Job drawing, mm, ordinate dimensions from the low corner. One solid piece. A direction names the side the tool comes from. Round coordinates to 2 decimals unless told otherwise and drop trailing zeros. Write each loop counter-clockwise with the first axis right and the second up, starting at its lowest first coordinate (ties: lowest second). Pieces come first, ordered by that corner, then holes.
1) Pull direction Y, two halves, no side cores. Call the marked faces 1, 2 and 3: +Y half, -Y half, draft (parallel to the pull), parting line (faces both ways), or undercut.
2) Saw through at B-B (y = 15.5). Write the cut outline in (x, z) (1 decimal).
3) Flat gauge pins, fed straight in: pin 1 (1 mm diameter, centred on y = 21, z = 1, fed in from +X); pin 2 (3.5 mm diameter, centred on y = 12.5, z = 1.5, fed in from -X); pin 3 (1 mm diameter, centred on y = 14, z = 6.5, fed in from +X) (1 decimal). Where does each tip first touch, or does it go through?
4) Wall check: probe 1 along Z at (x, y) = (6, 22.5); probe 2 along X at (y, z) = (27.5, 2.25); probe 3 along Z at (x, y) = (2, 30) (1 decimal). Give the ranges that are in metal, low to high.
5) Saw through at A-A (z = 6). State how many separate pieces and enclosed holes the cut face has, plus the area to 3 significant figures.
6) Which spindle directions (+Z, -Z, +X, -X, +Y, -Y) get a long thin tool onto all of the face, cutting with end or side? Do the marked faces 4, 5, 6 and 7. Say none if no direction does.
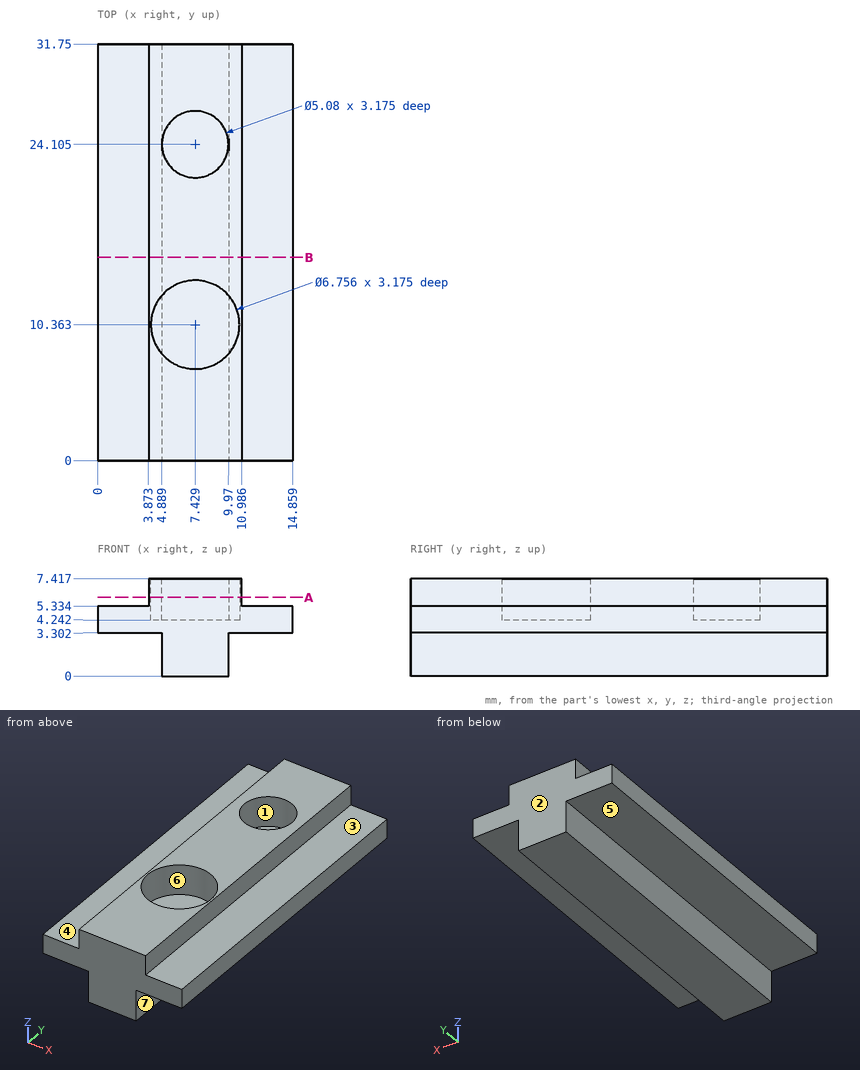
Evaluation:
1. face 1: undercut
1. face 2: +Y half
1. face 3: draft
2. outline: (0, 3.3) - (4.9, 3.3) - (4.9, 0) - (10, 0) - (10, 3.3) - (14.9, 3.3) - (14.9, 5.3) - (11, 5.3) - (11, 7.4) - (3.9, 7.4) - (3.9, 5.3) - (0, 5.3) - close
3. pin 1: stops at x = 9.97
3. pin 2: stops at x = 4.89
3. pin 3: stops at x = 11
4. probe 1: z = 0 to 4.24
4. probe 2: x = 4.89 to 9.97
4. probe 3: z = 3.3 to 5.3
5. separate pieces: 1
5. enclosed holes: 2
5. area: 170 mm2
6. face 4: +Z, -X, +Y, -Y
6. face 5: -Z, -X, +Y, -Y
6. face 6: +Z
6. face 7: -Z, +X, +Y, -Y
